Input: part model. Units: mm. Frame: model coordinates. A direction names the side the tool comes from. Give positions to 0.01 mm unless a question says otherwise; leave off trailing zeros. Loops run counter-clockwise (first coordinate to the right, second up) from the corner with the lowest first, then second, coordinate; pieces in that order, holes last. Notation, with made-up numbers: M 46.5,24.25 L 94.5,24.25 A7 ccw 94.5,33.25 Z; hole C 79.25,-10.5 d2. An arc over 180 degrees is marked long. Answer as a JSON object with one key per item and string values. Group by question number.
1) Ray query, L1, parallel to X at y = 0, z = 10.75; L2, parallel to Z at x = -34, y = 4; L3, parallel to Y at x = 0, z = 16.35. Return the intervals inside material, ascending.
2) Section query B-B on z = 2. Return loops of the section in (x, y).
3) Draft query along X for faces 1 (the flat face through (0, -31.177, 25)), 2 (the cylindrical face through (23.31, 7.34, 13.48)), 3 (the flat face through (-30.893, -17.505, 16.479)). Return one class per face: +X half, -X half, draft (parallel to the pull), parting line (faces both ways), or undercut.
4) Access query for faces 4 (the flat face through (-15, 24, 21)), 5 (the flat face through (0, 31.177, 25)), 6 (the flat face through (30.61, -18, 16.48)), 7 (the flat face through (-27.88, -15.8, 28.48)). Directions: +Z, -Z, +X, -X, +Y, -Y. A direction counts if a zero-diameter tool reaches every point of the face in a straight line with its end or side. Return the directions, or none.
5) Section query C-C on x = -34.5. Return loops of the section in (y, z), plus the area to 3 significant figures.
6) Section query A-A on z = 13. Return loops of the section in (x, y).
7) First-contact query: P1, Ø2.5, axis at x = -6.5, z = 14, coming from the +Y side; P2, Ø12, axis at x = -15, y = 10.5, coming from the +Z side; P3, Ø3, axis at x = 26, z = 4.5, coming from the -Y side (3 decimals). Flat tips, straight axial feed; report the tip coordinate or a pass-through.
from build123d import *

# Parameters (mm, degrees)
PAD_DEPTH    = 9
SKETCH001_W  = 26.1
SKETCH001_H  = 34.4
POCKET_DEPTH = 3
SKETCH002_R  = 22.22
PAD001_DEPTH = 3
SKETCH003_R  = 24.44
PAD002_DEPTH = 3
SKETCH004_R  = 26.6
PAD003_DEPTH = 3
SKETCH005_R  = 28
PAD004_DEPTH = 3
SKETCH006_R  = 29
PAD005_DEPTH = 3
SKETCH007_R  = 29
PAD006_DEPTH = 3
SKETCH008_R  = 29
PAD007_DEPTH = 3


with BuildPart() as part:
    # Sketch → Pad (new body)
    with BuildSketch(Plane.XY):
        Polygon((44, 0), (22, 38.105118), (-22, 38.105118), (-44, 0), (-22, -38.105118), (22, -38.105118), align=None)
    extrude(amount=PAD_DEPTH)

    # Sketch001 (on Face8 of Pad) → Pocket (cut)
    with BuildSketch(Plane.XY.offset(9)):
        with Locations((0, -13.905118)):
            Rectangle(SKETCH001_W, SKETCH001_H)
    extrude(amount=-POCKET_DEPTH, mode=Mode.SUBTRACT)

    # Sketch002 (on Face5 of Pocket) → Pad001 (join)
    with BuildSketch(Plane.XY.offset(9)):
        Polygon((22, 38.105118), (-22, 38.105118), (-44, 0), (-22, -38.105118), (22, -38.105118), (44, 0), align=None)
        Circle(SKETCH002_R, mode=Mode.SUBTRACT)
    extrude(amount=PAD001_DEPTH)

    # Sketch003 (on Face14 of Pad001) → Pad002 (join)
    with BuildSketch(Plane.XY.offset(12)):
        Polygon((40, 0), (20, 34.641016), (-20, 34.641016), (-40, 0), (-20, -34.641016), (20, -34.641016), align=None)
        Circle(SKETCH003_R, mode=Mode.SUBTRACT)
    extrude(amount=PAD002_DEPTH)

    # Sketch004 (on Face21 of Pad002) → Pad003 (join)
    with BuildSketch(Plane.XY.offset(15)):
        Polygon((41, 0), (20.5, 35.507042), (-20.5, 35.507042), (-41, 0), (-20.5, -35.507042), (20.5, -35.507042), align=None)
        Circle(SKETCH004_R, mode=Mode.SUBTRACT)
    extrude(amount=PAD003_DEPTH)

    # Sketch005 (on Face28 of Pad003) → Pad004 (join)
    with BuildSketch(Plane.XY.offset(18)):
        Polygon((19, 32.908965), (-19, 32.908965), (-38, 0), (-19, -32.908965), (19, -32.908965), (38, 0), align=None)
        Circle(SKETCH005_R, mode=Mode.SUBTRACT)
    extrude(amount=PAD004_DEPTH)

    # Sketch006 (on Face35 of Pad004) → Pad005 (join)
    with BuildSketch(Plane.XY.offset(21)):
        Polygon((39, 0), (19.5, 33.774991), (-19.5, 33.774991), (-39, 0), (-19.5, -33.774991), (19.5, -33.774991), align=None)
        Circle(SKETCH006_R, mode=Mode.SUBTRACT)
    extrude(amount=PAD005_DEPTH)

    # Sketch007 (on Face42 of Pad005) → Pad006 (join)
    with BuildSketch(Plane.XY.offset(24)):
        Polygon((36, 0), (18, 31.176915), (-18, 31.176915), (-36, 0), (-18, -31.176915), (18, -31.176915), align=None)
        Circle(SKETCH007_R, mode=Mode.SUBTRACT)
    extrude(amount=PAD006_DEPTH)

    # Sketch008 (on Face49 of Pad006) → Pad007 (join)
    with BuildSketch(Plane.XY.offset(27)):
        Polygon((37, 0), (18.5, 32.04294), (-18.5, 32.04294), (-37, 0), (-18.5, -32.04294), (18.5, -32.04294), align=None)
        Circle(SKETCH008_R, mode=Mode.SUBTRACT)
    extrude(amount=PAD007_DEPTH)


solid = part.part
Output:
{
 "1": {"L1": "x = -44 to -22.22, 22.22 to 44", "L2": "z = 0 to 24, 27 to 30", "L3": "y = -35.51 to -26.6, 26.6 to 35.51"},
 "2": {"outline": "M -44,0 L -22,-38.11 L 22,-38.11 L 44,0 L 22,38.11 L -22,38.11 Z"},
 "3": {"face 1": "draft", "face 2": "undercut", "face 3": "-X half"},
 "4": {"face 4": "+Z", "face 5": "+X, -X, +Y", "face 6": "+Z, +X, -Y", "face 7": "+Z, -X, -Y"},
 "5": {"outline": "M -16.45,0 L 16.45,0 L 16.45,12 L 9.53,12 L 9.53,15 L 11.26,15 L 11.26,18 L 6.06,18 L 6.06,21 L 7.79,21 L 7.79,24 L 2.6,24 L 2.6,27 L 4.33,27 L 4.33,30 L -4.33,30 L -4.33,27 L -2.6,27 L -2.6,24 L -7.79,24 L -7.79,21 L -6.06,21 L -6.06,18 L -11.26,18 L -11.26,15 L -9.53,15 L -9.53,12 L -16.45,12 Z", "area": "644 mm^2"},
 "6": {"outline": "M -40,0 L -20,-34.64 L 20,-34.64 L 40,0 L 20,34.64 L -20,34.64 Z; hole C 0,0 d48.88"},
 "7": {"P1": "stops at y = 35.51", "P2": "stops at z = 12", "P3": "stops at y = -33.775"}
}
